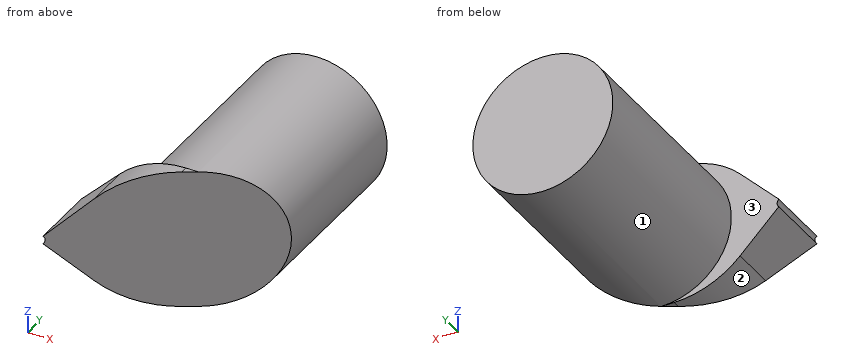
```python
from build123d import *

# Parameters (mm, degrees)
BOSS_EXTRUDE1_DEPTH     = 600
CUT_EXTRUDE1_DEPTH      = 743.024258364
CUT_EXTRUDE1_DEPTH_BACK = 743.024258364
CUT_EXTRUDE2_START      = -450
CUT_EXTRUDE2_DEPTH      = 450
FILLET1_R               = 200


with BuildPart() as part:
    # Sketch1 → Boss-Extrude1 (new body)
    with BuildSketch(Plane(origin=(0, 0, 0), x_dir=(1, 0, 0), z_dir=(0, 1, 0))):
        with BuildLine():
            Line((8.485281374, -8.485281374), (150, -150))
            Line((150, -150), (260, -150))
            ThreePointArc((260, -150), (410, 0), (260, 150))
            Line((260, 150), (150, 150))
            Line((150, 150), (8.485281374, 8.485281374))
            ThreePointArc((8.485281374, 8.485281374), (12, 0), (8.485281374, -8.485281374))
        make_face()
    extrude(amount=BOSS_EXTRUDE1_DEPTH)

    # Sketch2 → Cut-Extrude1 (cut, two sides: drawn at the far end of the back side and taken through both)
    with BuildSketch(Plane.XY.offset(-CUT_EXTRUDE1_DEPTH_BACK)):
        Polygon((0, 0), (410, 236.713610368), (410, 0), align=None)
    extrude(amount=CUT_EXTRUDE1_DEPTH + CUT_EXTRUDE1_DEPTH_BACK, mode=Mode.SUBTRACT)

    # Sketch3 → Cut-Extrude2 (cut)
    with BuildSketch(Plane(origin=(0, 600, 0), x_dir=(1, 0, 0), z_dir=(0, 1, 0)).offset(CUT_EXTRUDE2_START)):
        with BuildLine():
            Line((0, 0), (150, 150))
            Line((150, 150), (260, 150))
            ThreePointArc((260, 150), (110, 0), (260, -150))
            Line((260, -150), (150, -150))
            Line((150, -150), (0, 0))
        make_face()
    extrude(amount=CUT_EXTRUDE2_DEPTH, mode=Mode.SUBTRACT)

    # Fillet1
    fillet1_edges = [part.edges().sort_by_distance(p)[0] for p in [
        (150, 118.301270189, 150),
        (150, 118.301270189, -150),
    ]]
    fillet(fillet1_edges, radius=FILLET1_R)


solid = part.part
```
Build history of the part. All positions in model axes, mm. Face numbers are marked on the shaded views. A direction names the side the tool comes from. Round coordinates to 2 decimals unless told otherwise and drop trailing zeros. Write each loop counter-clockwise with the first axis right and the second up, starting at its lowest first coordinate (ties: lowest second). Pieces come first, ordered by that corner, then holes.
1) Band-saw the part on C-C, the plane y = 99.5. List the corners of the cut face in (x, z), and give its area (3 significant figures).
2) Band-saw the part on A-A, the plane x = 160. List the corners of the cut face in (y, z).
3) Pin check, flat tips, straight feed: pin 1 (1.5 mm diameter, centred on y = 383.5, z = 29.5, fed in from +X); pin 2 (1 mm diameter, centred on x = 278.5, y = 278, fed in from -Z); pin 3 (5 mm diameter, centred on y = 449, z = 80.5, fed in from +X). Stop position of each tip, or through.
4) 3-axis set-ups, long thin cutter, end or side, ignore diameter. For the marked faces 1, 2 and 3: which of +Z, -Z, +X, -X, +Y, -Y reach the whole face in a straight line?
5) Drill centre lines: probe 1 along X at (y, z) = (473, 2); probe 2 along X at (y, z) = (243, 25); probe 3 along Z at (x, y) = (294, 392). Where is each one in solid material? Low to high.
6) Band-saw the part on D-D, the plane y = 526. List the corners of the cut face in (x, z).
7) Band-saw the part on B-B, the plane z = 0. List the corners of the cut face in (x, y), and give its area (3 significant figures).
Ans:
1. outline: (8.49, -8.49) - (91.42, -91.42) arc R200 ccw to (172.34, -140.63) - (172.34, 140.63) arc R200 ccw to (91.42, 91.42) - (8.49, 8.49) arc R12 cw to start
1. area: 27,700 mm2
2. outline: (92.38, -136.26) - (150, -136.26) - (150, -111.8) - (600, -111.8) - (600, 111.8) - (150, 111.8) - (150, 136.26) - (92.38, 136.26) - close
3. pin 1: stops at x = 407.22
3. pin 2: stops at z = -148.92
3. pin 3: stops at x = 388.12
4. face 1: +Y
4. face 2: -Z, -X, +Y, -Y
4. face 3: -X, +Y
5. probe 1: x = 110.01 to 409.99
5. probe 2: x = 112.1 to 407.9
5. probe 3: z = -146.1 to 146.1
6. outline: circle Ø300 at (260, 0)
7. outline: (12, 6.93) - (410, 236.71) - (410, 600) - (110, 600) - (110, 150) - (12, 150) - close
7. area: 146,000 mm2
